The drawing under review shows one solid part. Ordinate dimensions are in mm from its lowest x, y, z. Give positions to 0.01 mm unless a question says otherwise; leave off trailing zeros. Write each loop counter-clockwise with the first axis right and the second up, starting at its lowest first coordinate (ties: lowest second). Pieces come first, ordered by that corner, then holes. Notation, with made-up numbers: (9, -28) -> (59, -28) arc R22 ccw to (59, -21) -> close; hole circle Ø11 at (56.5, 52). An arc over 180 degrees is marked (long way). Use CSV: the item, a comma, the result in double quotes.
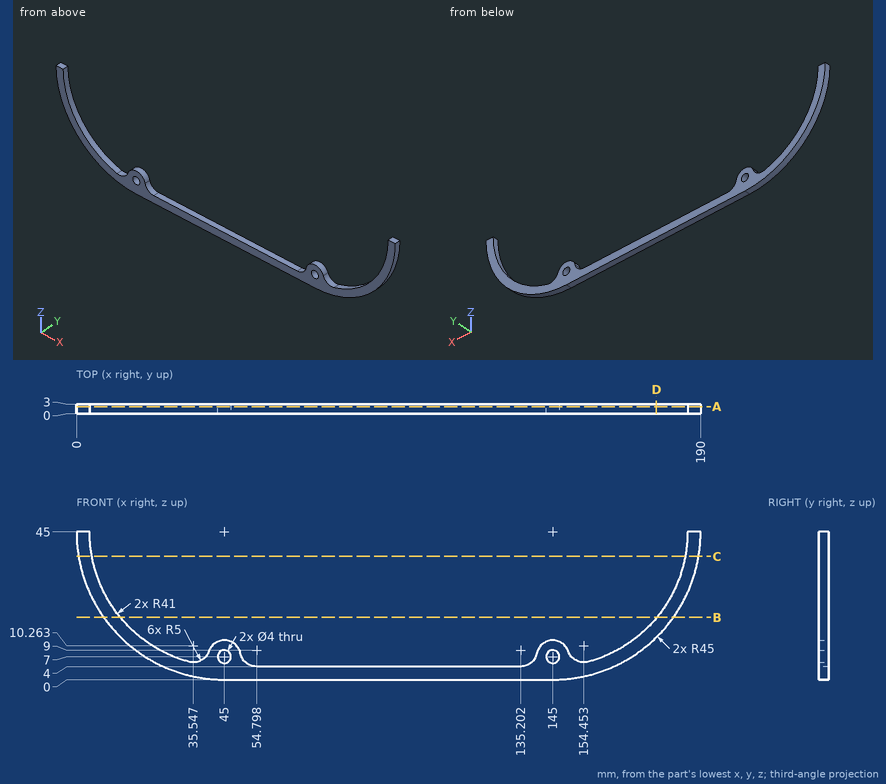
(1) Take a section at B-B (z = 19). Write out the cut boundary in (x, y).
Established:
outline,"(8.27, 0) -> (13.3, 0) -> (13.3, 3) -> (8.27, 3) -> close; (176.7, 0) -> (181.73, 0) -> (181.73, 3) -> (176.7, 3) -> close"
(2) For line 1 along Z through (x, y) = (45, 2.05); line 2 along Z through (x, y) = (120, 1.1); line 3 along X through (y, z) = (1.55, 34.5), list the stretches that pass through material, from the lowest coordinate up. Write a range as [from, to].
Established:
line 1,"z = [0, 5], [9, 12]"
line 2,"z = [0, 4]"
line 3,"x = [1.24, 5.37], [184.63, 188.76]"
(3) Take a section at C-C (z = 37.5). Write out the cut boundary in (x, y).
Established:
outline,"(0.63, 0) -> (4.69, 0) -> (4.69, 3) -> (0.63, 3) -> close; (185.31, 0) -> (189.37, 0) -> (189.37, 3) -> (185.31, 3) -> close"
(4) Clearance check with flat-ended pins moving along their axes: pin 1 (3 mm diameter, centred on x = 145, z = 7, fed in from +Y); pin 2 (1.5 mm diameter, centred on x = 139.5, z = 6, fed in from -Y). State where each tip first meets the part, or that it passes through.
Established:
pin 1,"passes through"
pin 2,"stops at y = 0"
(5) Take a section at D-D (x = 176.5). Write out the cut boundary in (y, z).
Established:
outline,"(0, 12.86) -> (3, 12.86) -> (3, 18.76) -> (0, 18.76) -> close"
(6) Take a section at A-A (y = 2.2). Write out the cut boundary in (x, z) (1 decimal), then the cut area to 3 significant figures.
Established:
outline,"(0, 45) arc R45 ccw to (45, 0) -> (145, 0) arc R45 ccw to (190, 45) -> (186, 45) arc R41 cw to (155.8, 5.4) arc R5 cw to (149.7, 8.6) arc R5 ccw to (140.1, 8) arc R5 cw to (135.2, 4) -> (54.8, 4) arc R5 cw to (49.9, 8) arc R5 ccw to (40.3, 8.6) arc R5 cw to (34.2, 5.4) arc R41 cw to (4, 45) -> close; hole circle Ø4 at (45, 7); hole circle Ø4 at (145, 7)"
area,"1,070 mm2"
